```python
from build123d import *

# Parameters (mm, degrees)
SKIZZE1_W                       = 271
SKIZZE1_H                       = 70
AUFSATZ_LINEAR_AUSTRAGEN1_DEPTH = 5
SKIZZE2_W                       = 72
SKIZZE2_H                       = 70
SCHNITT_LINEAR_AUSTRAGEN1_DEPTH = 3
SKIZZE3_R                       = 4
SCHNITT_LINEAR_AUSTRAGEN2_DEPTH = 10
SKIZZE4_R                       = 2.5
SCHNITT_LINEAR_AUSTRAGEN3_DEPTH = 10
SKIZZE5_R                       = 2.5
SCHNITT_LINEAR_AUSTRAGEN4_DEPTH = 10
SKIZZE6_R                       = 2
SCHNITT_LINEAR_AUSTRAGEN5_DEPTH = 10
SKIZZE7_R                       = 19.0625
SKIZZE7_R_2                     = 2.5
SCHNITT_LINEAR_AUSTRAGEN6_DEPTH = 10
SKIZZE8_R                       = 4
SCHNITT_LINEAR_AUSTRAGEN7_DEPTH = 10
SKIZZE9_R                       = 2
SCHNITT_LINEAR_AUSTRAGEN8_DEPTH = 10


with BuildPart() as part:
    # Skizze1 → Aufsatz-Linear austragen1 (new body)
    with BuildSketch(Plane.XY):
        with Locations((135.5, 35)):
            Rectangle(SKIZZE1_W, SKIZZE1_H)
    extrude(amount=AUFSATZ_LINEAR_AUSTRAGEN1_DEPTH)

    # Skizze2 → Schnitt-Linear austragen1 (cut)
    with BuildSketch(Plane.XY.offset(5)):
        with Locations((190.5, 35)):
            Rectangle(SKIZZE2_W, SKIZZE2_H)
    extrude(amount=-SCHNITT_LINEAR_AUSTRAGEN1_DEPTH, mode=Mode.SUBTRACT)

    # Skizze3 → Schnitt-Linear austragen2 (cut)
    with BuildSketch(Plane(origin=(0, 0, 0), x_dir=(-1, 0, 0), z_dir=(0, 0, -1))):
        with Locations((-160.5, 37)):
            Circle(SKIZZE3_R)
        with Locations((-220.5, 37)):
            Circle(SKIZZE3_R)
        with Locations((-220.5, 7)):
            Circle(SKIZZE3_R)
        with Locations((-160.5, 7)):
            Circle(SKIZZE3_R)
    extrude(amount=-SCHNITT_LINEAR_AUSTRAGEN2_DEPTH, mode=Mode.SUBTRACT)

    # Skizze4 → Schnitt-Linear austragen3 (cut)
    with BuildSketch(Plane(origin=(0, 0, 0), x_dir=(-1, 0, 0), z_dir=(0, 0, -1))):
        with Locations((-234.5, 23.5)):
            Circle(SKIZZE4_R)
        with Locations((-266.5, 23.5)):
            Circle(SKIZZE4_R)
    extrude(amount=-SCHNITT_LINEAR_AUSTRAGEN3_DEPTH, mode=Mode.SUBTRACT)

    # Skizze5 → Schnitt-Linear austragen4 (cut)
    with BuildSketch(Plane(origin=(0, 0, 0), x_dir=(-1, 0, 0), z_dir=(0, 0, -1))):
        with Locations((-36.5, 23.5)):
            Circle(SKIZZE5_R)
        with Locations((-4.5, 23.5)):
            Circle(SKIZZE5_R)
    extrude(amount=-SCHNITT_LINEAR_AUSTRAGEN4_DEPTH, mode=Mode.SUBTRACT)

    # Skizze6 → Schnitt-Linear austragen5 (cut)
    with BuildSketch(Plane(origin=(0, 0, 0), x_dir=(-1, 0, 0), z_dir=(0, 0, -1))):
        with Locations((-10, 60)):
            Circle(SKIZZE6_R)
        with Locations((-50, 60)):
            Circle(SKIZZE6_R)
        with Locations((-160.5, 60)):
            Circle(SKIZZE6_R)
        with Locations((-220.5, 60)):
            Circle(SKIZZE6_R)
        with Locations((-261, 60)):
            Circle(SKIZZE6_R)
    extrude(amount=-SCHNITT_LINEAR_AUSTRAGEN5_DEPTH, mode=Mode.SUBTRACT)

    # Skizze7 → Schnitt-Linear austragen6 (cut)
    with BuildSketch(Plane(origin=(0, 0, 0), x_dir=(-1, 0, 0), z_dir=(0, 0, -1))):
        with Locations((-119.5, 32)):
            Circle(SKIZZE7_R)
        with Locations((-95.93, 8.43)):
            Circle(SKIZZE7_R_2)
        with Locations((-143.07, 8.43)):
            Circle(SKIZZE7_R_2)
        with Locations((-95.93, 55.57)):
            Circle(SKIZZE7_R_2)
        with Locations((-143.07, 55.57)):
            Circle(SKIZZE7_R_2)
    extrude(amount=-SCHNITT_LINEAR_AUSTRAGEN6_DEPTH, mode=Mode.SUBTRACT)

    # Skizze8 → Schnitt-Linear austragen7 (cut)
    with BuildSketch(Plane(origin=(0, 0, 0), x_dir=(-1, 0, 0), z_dir=(0, 0, -1))):
        with Locations((-59.5, 40)):
            Circle(SKIZZE8_R)
    extrude(amount=-SCHNITT_LINEAR_AUSTRAGEN7_DEPTH, mode=Mode.SUBTRACT)

    # Skizze9 → Schnitt-Linear austragen8 (cut)
    with BuildSketch(Plane.XY.offset(5)):
        with Locations((75, 60)):
            Circle(SKIZZE9_R)
    extrude(amount=-SCHNITT_LINEAR_AUSTRAGEN8_DEPTH, mode=Mode.SUBTRACT)


solid = part.part
```
Geometry check sheet. Reference: the model listing, model coordinates, mm. A direction names the side the tool comes from. Coordinates: 2 decimals unless noted, no trailing zeros. Order: outer loops, then holes, each group sorted by start corner. A loop starts at its lowest first (then second) coordinate and runs counter-clockwise, first axis right, second up. Notation, with made-up numbers: M 31,66 L 35,66 A38 ccw 35,105 Z; hole C 87.5,46 d1. An arc over 180 degrees is marked long. Answer as a JSON object with one key per item and string values.
Q1. Depth check by flat-ended pin: pin 1 Ø7 at (x, y) = (160.5, 37) entering from +Z; pin 2 Ø4 at (x, y) = (224, 15.5) entering from +Z. Enter the tip coordinate at first touch or a pass-through.
Results are:
{"pin 1": "passes through", "pin 2": "stops at z = 2"}
Q2. Scan lines: line 1 (X direction, y = 55.5, z = 0.7); line 2 (Y direction, x = 95.93, z = 1.6); line 3 (Y direction, x = 261, z = 1.55). Record each from-to range of solid material in increasing order.
Results are:
{"line 1": "x = 0 to 93.43, 98.43 to 140.57, 145.57 to 271", "line 2": "y = 0 to 5.93, 10.93 to 53.07, 58.07 to 70", "line 3": "y = 0 to 58, 62 to 70"}
Q3. Cross-section at D-D on x = 116.5. Record the cut outline in (y, z).
Results are:
{"outline": "M 0,0 L 13.18,0 L 13.18,5 L 0,5 Z; M 50.82,0 L 70,0 L 70,5 L 50.82,5 Z"}
Q4. Cross-section at C-C on y = 29.5. Record the cut outline in (x, z), and give its area (3 significant figures).
Results are:
{"outline": "M 0,0 L 100.6,0 L 100.6,5 L 0,5 Z; M 138.4,0 L 271,0 L 271,5 L 226.5,5 L 226.5,2 L 154.5,2 L 154.5,5 L 138.4,5 Z", "area": "950 mm²"}
Q5. Cross-section at A-A on z = 3.5. Give the number of separate pieces and of enclosed holes in the cut face, and give its area (3 significant figures).
Results are:
{"separate pieces": "2", "enclosed holes": "14", "area": "12,500 mm²"}
Q6. Release check for a two-part mould opening along X. For faces 3 (the flat face through (271, 35, 2)), 4 (the flat face through (76, 35, 5)), 5 (the cylindrical face through (140.685, 56.321, 2.465)) record: released by +X, released by -X, zero draft, split by the parting line, or undercut.
Results are:
{"face 3": "released by +X", "face 4": "zero draft", "face 5": "undercut"}
Q7. Tool access check on faces 1 (the cylindrical face through (3.16, 25.61, 2.46)), 2 (the flat face through (190, 35, 2)). Record the directions out of +Z, -Z, +X, -X, +Y, -Y that give a thin tool (end or side, any length) a straight path to the whole face; none if there is none.
Results are:
{"face 1": "+Z, -Z", "face 2": "+Z, +Y, -Y"}
Q8. Cross-section at B-B on y = 55.57. Record the cut outline in (x, z), and give its area (3 significant figures).
Results are:
{"outline": "M 0,0 L 93.43,0 L 93.43,5 L 0,5 Z; M 98.43,0 L 140.57,0 L 140.57,5 L 98.43,5 Z; M 145.57,0 L 271,0 L 271,5 L 226.5,5 L 226.5,2 L 154.5,2 L 154.5,5 L 145.57,5 Z", "area": "1,090 mm²"}
